Verification items for the finished model (mm, model axes). Give positions to 0.01 mm unless a question says otherwise; leave off trailing zeros. Loops run counter-clockwise (first coordinate to the right, second up) from the corner with the lowest first, then second, coordinate; pieces in that order, holes last. Notation, with made-up numbers: (-19.75, 31) - (-8.75, 31) arc R23 cw to (-8.75, 67) - close; hole circle Ø7 at (19.25, 39.25). An arc over 180 degrees is marked (long way). Use one line per item in the form item = value.
```python
from build123d import *

# Parameters (mm, degrees)
F1_DEPTH = 3.2
F2_R     = 1
F3_DEPTH = 3.2


with BuildPart() as f1:
    # F0 (on Top) → F1 (new body)
    with BuildSketch(Plane.XY):
        with BuildLine():
            ThreePointArc((-115.903488, 49.952005), (-116.838218, 48.881038), (-117.175, 47.5))
            Line((-117.175, 47.5), (-117.175, -47.5))
            ThreePointArc((-117.175, -47.5), (-116.29632, -49.62132), (-114.175, -50.5))
            Line((-114.175, -50.5), (114.175, -50.5))
            ThreePointArc((114.175, -50.5), (115.081638, -50.359722), (115.903488, -49.952005))
            Line((115.903488, -49.952005), (0, 0))
            Line((0, 0), (-115.903488, 49.952005))
        make_face()
        with BuildLine():
            ThreePointArc((-114.175, 50.5), (-115.081638, 50.359722), (-115.903488, 49.952005))
            Line((-115.903488, 49.952005), (0, 0))
            Line((0, 0), (115.903488, -49.952005))
            ThreePointArc((115.903488, -49.952005), (116.838218, -48.881038), (117.175, -47.5))
            Line((117.175, -47.5), (117.175, 47.5))
            ThreePointArc((117.175, 47.5), (116.29632, 49.62132), (114.175, 50.5))
            Line((114.175, 50.5), (-68.531, 50.5))
            Line((-68.531, 50.5), (-68.531, 56.75))
            Line((-68.531, 56.75), (-86.311, 56.75))
            Line((-86.311, 56.75), (-86.311, 50.5))
            Line((-86.311, 50.5), (-114.175, 50.5))
        make_face()
    extrude(amount=F1_DEPTH)

    # F2 (on face) → F3 (cut)
    with BuildSketch(Plane.XY.offset(3.2)):
        with Locations((96.832131, -28.57509)):
            Circle(F2_R)
        with Locations((95.25071, 28.57509)):
            Circle(F2_R)
        with BuildLine():
            ThreePointArc((37.205863, -28.127877), (37.870537, -29.548339), (39.10029, -28.57509))
            ThreePointArc((39.10029, -28.57509), (38.330043, -27.601841), (37.205863, -28.127877))
        make_face()
        with BuildLine():
            ThreePointArc((-37.10029, -28.57509), (-37.127041, -28.345337), (-37.205863, -28.127877))
            ThreePointArc((-37.205863, -28.127877), (-39.073539, -28.804843), (-37.10029, -28.57509))
        make_face()
        with BuildLine():
            ThreePointArc((-37.10029, 28.57509), (-39.073539, 28.804843), (-37.205863, 28.127877))
            ThreePointArc((-37.205863, 28.127877), (-37.127041, 28.345337), (-37.10029, 28.57509))
        make_face()
        with BuildLine():
            ThreePointArc((39.10029, 28.57509), (37.870537, 29.548339), (37.205863, 28.127877))
            ThreePointArc((37.205863, 28.127877), (38.330043, 27.601841), (39.10029, 28.57509))
        make_face()
        with BuildLine():
            ThreePointArc((-0.894427, 9.972183), (-0.850651, 8.999239), (0, 8.52497))
            Line((0, 8.52497), (0, 9.52497))
            Line((0, 9.52497), (-0.894427, 9.972183))
        make_face()
        with BuildLine():
            Line((0, 9.52497), (0, 8.52497))
            ThreePointArc((0, 8.52497), (0.707107, 8.817863), (1, 9.52497))
            ThreePointArc((1, 9.52497), (0.973249, 9.754723), (0.894427, 9.972183))
            Line((0.894427, 9.972183), (0, 9.52497))
        make_face()
        with BuildLine():
            ThreePointArc((-0.894427, -9.972183), (0, -10.52497), (0.894427, -9.972183))
            Line((0.894427, -9.972183), (0, -9.52497))
            Line((0, -9.52497), (-0.894427, -9.972183))
        make_face()
        with BuildLine():
            Line((0, -9.52497), (0.894427, -9.972183))
            ThreePointArc((0.894427, -9.972183), (0.973249, -9.754723), (1, -9.52497))
            ThreePointArc((1, -9.52497), (0.707107, -8.817863), (0, -8.52497))
            Line((0, -8.52497), (0, -9.52497))
        make_face()
        with BuildLine():
            ThreePointArc((0, -8.52497), (-0.850651, -8.999239), (-0.894427, -9.972183))
            Line((-0.894427, -9.972183), (0, -9.52497))
            Line((0, -9.52497), (0, -8.52497))
        make_face()
        with BuildLine():
            ThreePointArc((0.894427, 9.972183), (0, 10.52497), (-0.894427, 9.972183))
            Line((-0.894427, 9.972183), (0, 9.52497))
            Line((0, 9.52497), (0.894427, 9.972183))
        make_face()
        with Locations((-95.24909, -28.57509)):
            Circle(F2_R)
        with Locations((-95.24909, 28.57509)):
            Circle(F2_R)
    extrude(amount=-F3_DEPTH, mode=Mode.SUBTRACT)


solid = f1.part
```
1. Scan lines: probe 1 along X at (y, z) = (28, 2.85) (3 decimals); probe 2 along Y at (x, z) = (5.5, 0.7); probe 3 along X at (y, z) = (51.5, 3.15). Record each from-to range of solid material in increasing order.
Result set:
probe_1 = -117.175 to -96.067, -94.431 to -38.918, -37.282 to 37.282, 38.918 to 94.433, 96.069 to 117.175
probe_2 = -50.5 to 50.5
probe_3 = -86.31 to -68.53
2. Depth check by flat-ended pin: pin 1 Ø3 at (x, y) = (38.1, 28.58) entering from -Z; pin 2 Ø1.6 at (x, z) = (39, 1.5) entering from +Y. Enter the tip coordinate at first touch or a pass-through.
Result set:
pin_1 = 0
pin_2 = 50.5
3. Section check A-A, the plane z = 1.5. State how many separate pieces and enclosed holes the cut face has, then the cut area to 3 significant figures.
Result set:
separate_pieces = 1
enclosed_holes = 10
area = 23,700 mm²
4. Section check B-B, the plane x = 80.5. Record the cut outline in (y, z), then the cut area to 3 significant figures.
Result set:
outline = (-50.5, 0) - (50.5, 0) - (50.5, 3.2) - (-50.5, 3.2) - close
area = 323 mm²
